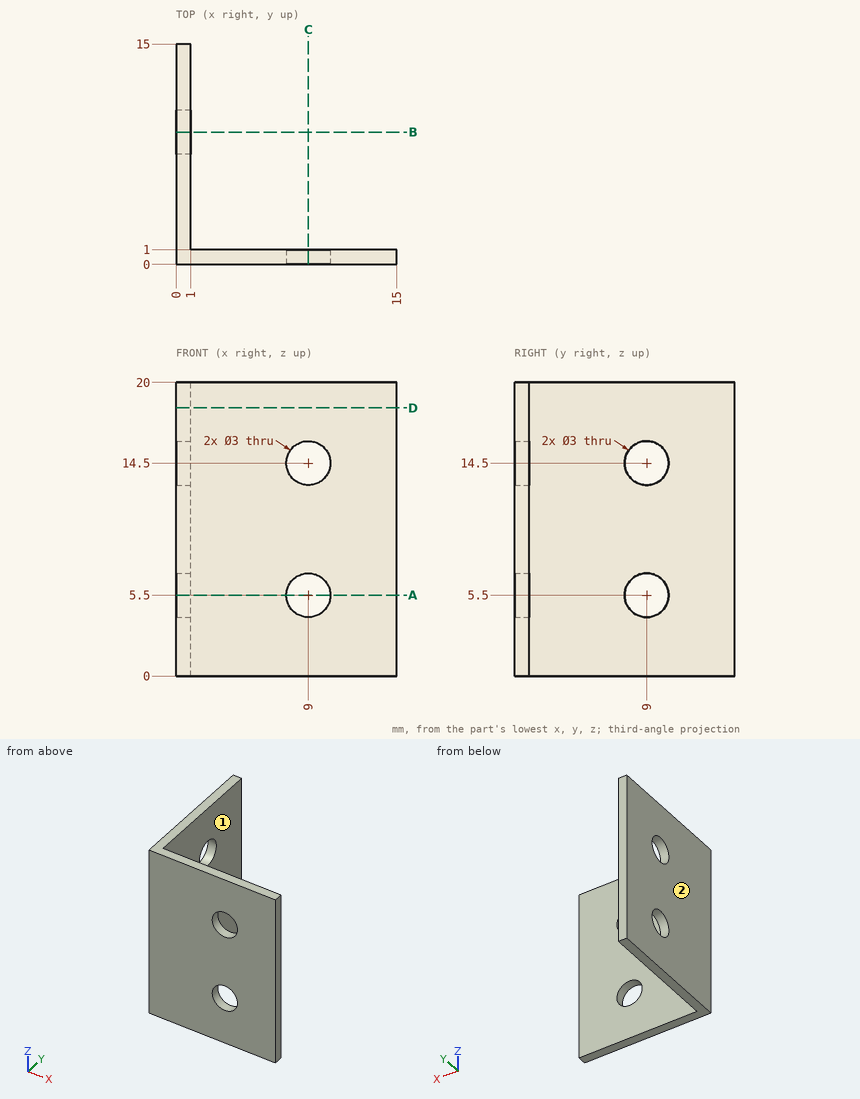
Answer from the drawing. Dimensions are ordinates in mm from the lowest x, y and z of the part. A direction names the side the tool comes from. Coordinates: 2 decimals unless noted, no trailing zeros. Loops run counter-clockwise (first coordinate to the right, second up) from the corner with the lowest first, then second, coordinate; pieces in that order, holes last.
1) Section A-A (z = 5.5) is taken. Give the vertices of the cut face in (x, y).
Results:
outline: (0, 0) - (7.5, 0) - (7.5, 1) - (1, 1) - (1, 7.5) - (0, 7.5) - close; (0, 10.5) - (1, 10.5) - (1, 15) - (0, 15) - close; (10.5, 0) - (15, 0) - (15, 1) - (10.5, 1) - close
2) Section B-B (y = 9) is taken. Give the vertices of the cut face in (x, z), plus the area to 3 significant figures.
Results:
outline: (0, 0) - (1, 0) - (1, 4) - (0, 4) - close; (0, 7) - (1, 7) - (1, 13) - (0, 13) - close; (0, 16) - (1, 16) - (1, 20) - (0, 20) - close
area: 14.0 mm2
3) Consider probe 1 along Z at (x, y) = (9, 0.8); probe 2 along X at (y, z) = (0.75, 14.5); probe 3 along Y at (x, z) = (3, 16). Determine where each line is inside the solid, lowest interval first.
Results:
probe 1: z = 0 to 4, 7 to 13, 16 to 20
probe 2: x = 0 to 7.5, 10.5 to 15
probe 3: y = 0 to 1
4) Flat-ended cylindrical pins translate along their axes: pin 1 (3 mm diameter, centred on x = 4, z = 4, fed in from +Y); pin 2 (3.5 mm diameter, centred on y = 9, z = 5.5, fed in from +X). Find the tip coordinate at first contact, or state that the pin passes through.
Results:
pin 1: stops at y = 1
pin 2: stops at x = 1
5) Section D-D (z = 18.25) is taken. Give the vertices of the cut face in (x, y).
Results:
outline: (0, 0) - (15, 0) - (15, 1) - (1, 1) - (1, 15) - (0, 15) - close
6) For the marked faces 1 and 2, determine the directions among +Z, -Z, +X, -X, +Y, -Y from which every point of the face is accessible in a straight line to the end or side of a thin tool.
Results:
face 1: +Z, -Z, +X, +Y
face 2: +Z, -Z, -X, +Y, -Y
